from build123d import *

# Parameters (mm, degrees)
BOSS_EXTRUDE1_DEPTH      = 0.94869
BOSS_EXTRUDE1_DEPTH_BACK = 0.94869
SKETCH4_R                = 2.8067
CUT_EXTRUDE1_DEPTH       = 1.94869
CUT_EXTRUDE1_DEPTH_BACK  = 1.94869
SKETCH5_R                = 4.2164
CUT_EXTRUDE2_DEPTH       = 2.89738
CUT_EXTRUDE2_TAPER       = 41


with BuildPart() as part:
    # Sketch3 → Boss-Extrude1 (new body, two sides)
    with BuildSketch(Plane.XY) as boss_extrude1_sk:
        Polygon((-44.45, 44.45), (-28.575, 44.45), (-28.575, -28.575), (44.45, -28.575), (44.45, -44.45), (-44.45, -44.45), align=None)
    extrude(amount=BOSS_EXTRUDE1_DEPTH)
    extrude(boss_extrude1_sk.sketch, amount=-BOSS_EXTRUDE1_DEPTH_BACK)

    # Sketch4 → Cut-Extrude1 (cut, two sides)
    with BuildSketch(Plane.XY) as cut_extrude1_sk:
        with Locations((-36.5125, 30.1498)):
            Circle(SKETCH4_R)
        with Locations((-36.5125, -13.5128)):
            Circle(SKETCH4_R)
        with Locations((-13.5128, -36.5125)):
            Circle(SKETCH4_R)
        with Locations((30.1498, -36.5125)):
            Circle(SKETCH4_R)
    extrude(amount=CUT_EXTRUDE1_DEPTH, mode=Mode.SUBTRACT)
    extrude(cut_extrude1_sk.sketch, amount=-CUT_EXTRUDE1_DEPTH_BACK, mode=Mode.SUBTRACT)

    # Sketch5 → Cut-Extrude2 (cut, through all)
    with BuildSketch(Plane.XY.offset(0.94869)):
        with Locations((-36.5125, 30.1498)):
            Circle(SKETCH5_R)
        with Locations((-36.5125, -13.5128)):
            Circle(SKETCH5_R)
        with Locations((-13.5128, -36.5125)):
            Circle(SKETCH5_R)
        with Locations((30.1498, -36.5125)):
            Circle(SKETCH5_R)
    extrude(amount=-CUT_EXTRUDE2_DEPTH, taper=CUT_EXTRUDE2_TAPER, mode=Mode.SUBTRACT)


solid = part.part
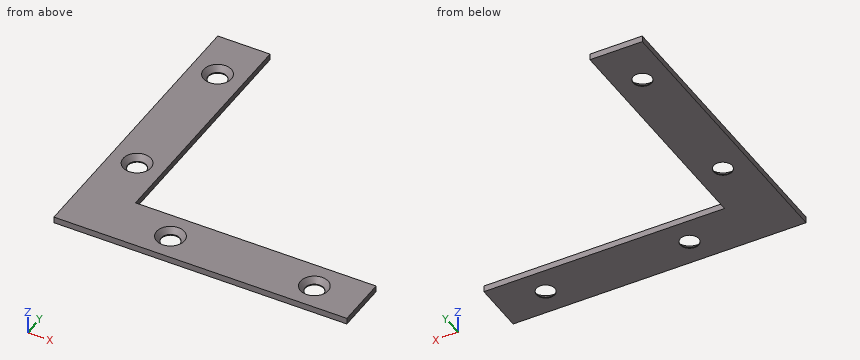
Model file for the job. Use its own axes, mm. Round coordinates to 2 decimals unless told otherwise and drop trailing zeros. Loops run counter-clockwise (first coordinate to the right, second up) from the corner with the lowest first, then second, coordinate; pieces in that order, holes last. Notation, with made-up numbers: (63, 42) -> (86, 42) arc R11 cw to (86, 60) -> close; hole circle Ø5 at (76.25, -26). An arc over 180 degrees is marked (long way). Answer as CSV lines item,"result". Start each with the question number.
1) Pin check, flat tips, straight feed: P1, Ø0.6, axis at y = -10, z = 0.5, coming from the +X side (3 decimals); P2, Ø7.5, axis at x = 30.15, y = -36.51, coming from the -Z side. Stop position of each tip, or through.
2) Probe line 1 along X through (y, z) = (-38.5, 0.05); line 2 along Y through (x, z) = (-36.5, -0.5); line 3 along Y through (x, z) = (-35, -0.3). List the from-to ranges inside material, lowest first.
3) Slice it at A-A (z = 0). State how many separate pieces and enclosed holes the cut face has, plus the area to 3 significant figures.
4) Slice it at B-B (x = 39). List the corners of the cut face in (y, z) (3 decimals), plus the area to 3 significant figures.
Filled in:
1,P1,"stops at x = -28.575"
1,P2,"stops at z = -0.95"
2,line 1,"x = -44.45 to -16.31, -10.71 to 27.35, 32.95 to 44.45"
2,line 2,"y = -44.45 to -16.47, -10.56 to 27.19, 33.11 to 44.45"
2,line 3,"y = -44.45 to -16.25, -10.77 to 27.41, 32.89 to 44.45"
3,separate pieces,"1"
3,enclosed holes,"4"
3,area,"2,430 mm2"
4,outline,"(-44.45, -0.949) -> (-28.575, -0.949) -> (-28.575, 0.949) -> (-44.45, 0.949) -> close"
4,area,"30.1 mm2"
